Build history of the part. All positions in model axes, mm. A direction names the side the tool comes from. Give positions to 0.01 mm unless a question says otherwise; leave off trailing zeros. Order: outer loops, then holes, each group sorted by start corner. A loop starts at its lowest first (then second) coordinate and runs counter-clockwise, first axis right, second up. Notation, with made-up numbers: M 65.5,43.25 L 95.5,43.25 A16 cw 95.5,59.25 Z; hole C 44,39 d4. An arc over 180 degrees is marked long. Use CSV: the item, a comma, the result in double quotes. Start each with the question number.
Item 1: Two-plate mould, pull along Z, no slides. Class faces 4 (the flat face through (-10.433, 25, 3)), 5 (the flat face through (-12.433, 26, 2)), 6 (the cylindrical face through (-9.357, 35.21, 0.994)), 7 (the flat face through (11, 68, -1.834)): pulls with the +Z half, pulls with the -Z half, needs draft (parallel to the pull), parting line crosses it, or undercut.
Item 2: Which spindle directions (+Z, -Z, +X, -X, +Y, -Y) get a long thin tool onto all of the face, cutting with end or side? Do faces 1 (the flat face through (-2.933, 79, -12)), 2 (the cylindrical face through (2.27, 72.71, 10.75)), 3 (the flat face through (2.067, 79, -12)). Say none if no direction does.
Item 3: Band-saw the part on D-D on z = -11. Write the cut outline in (x, y), plus the area to 3 significant figures.
Item 4: Band-saw the part on A-A on y = 32. Write the cut outline in (x, z).
Item 5: Wall check: line 1 along X through (y, z) = (19, 3.5); line 2 along Z through (x, y) = (8.75, 30); line 3 along Z through (x, y) = (4.5, 45.5). Give the ranges that are in metal, low to high.
Item 6: Band-saw the part on B-B on y = 17.5. Write the cut outline in (x, z).
Item 7: Band-saw the part on C-C on x = -4.5. Write the cut outline in (y, z).
Item 8: Pin check, flat tips, straight feed: P1, Ø3, axis at x = 6, z = 8.5, coming from the -Y side; P2, Ø2, axis at x = 7.5, z = -8.5, coming from the -Y side; P3, Ø7, axis at x = 0.5, z = 1.5, coming from the -Y side; P4, Ø1.5, axis at y = 73.5, z = 2.5, coming from the +X side. Stop position of each tip, or through.
from build123d import *

# Parameters (mm, degrees)
SKETCH1_W            = 24
SKETCH1_H            = 24
SKETCH1_W_2          = 20
SKETCH1_H_2          = 20
BOSS_EXTRUDE1_DEPTH  = 50
FILLET1_R            = 1
FILLET2_R            = 1
BOSS_EXTRUDE7_START  = 2
BOSS_EXTRUDE7_DEPTH  = 2
SKETCH9_R            = 9
BOSS_EXTRUDE9_DEPTH  = 30
SKETCH10_R           = 7
CUT_EXTRUDE1_DEPTH   = 34
SKETCH11_R           = 9
SKETCH11_R_2         = 7
BOSS_EXTRUDE10_DEPTH = 40
BOSS_EXTRUDE12_DEPTH = 1
FILLET3_R            = 1
SKETCH15_R           = 9
BOSS_EXTRUDE13_DEPTH = 2
BOSS_EXTRUDE15_DEPTH = 1
FILLET5_R            = 1
SKETCH18_W           = 5
SKETCH18_H           = 5
BOSS_EXTRUDE16_DEPTH = 1


with BuildPart() as part:
    # Sketch1 → Boss-Extrude1 (new body)
    with BuildSketch(Plane(origin=(0, 0, 0), x_dir=(1, 0, 0), z_dir=(0, 1, 0))):
        with Locations((-0.433212996, -2.166064982)):
            Rectangle(SKETCH1_W, SKETCH1_H)
        with Locations((-0.433212996, -2.166064982)):
            Rectangle(SKETCH1_W_2, SKETCH1_H_2, mode=Mode.SUBTRACT)
    extrude(amount=BOSS_EXTRUDE1_DEPTH)

    # Fillet1
    fillet1_edges = [part.edges().sort_by_distance(p)[0] for p in [
        (-10.433212996, 25, -7.833935018),
        (11.566787004, 25, -9.833935018),
        (11.566787004, 25, 14.166064982),
        (-12.433212996, 25, 14.166064982),
    ]]
    fillet(fillet1_edges, radius=FILLET1_R)

    # Fillet2
    fillet2_edges = [part.edges().sort_by_distance(p)[0] for p in [
        (-12.433212996, 25, -9.833935018),
    ]]
    fillet(fillet2_edges, radius=FILLET2_R)

    # Sketch8 → Boss-Extrude7 (add)
    with BuildSketch(Plane(origin=(0, 50, 0), x_dir=(1, 0, 0), z_dir=(0, 1, 0)).offset(BOSS_EXTRUDE7_START)):
        with BuildLine():
            Line((10.566787004, 9.833935018), (-11.433212996, 9.833935018))
            ThreePointArc((-11.433212996, 9.833935018), (-12.140319778, 9.541041799), (-12.433212996, 8.833935018))
            Line((-12.433212996, 8.833935018), (-12.433212996, -13.166064982))
            ThreePointArc((-12.433212996, -13.166064982), (-12.140319778, -13.873171763), (-11.433212996, -14.166064982))
            Line((-11.433212996, -14.166064982), (10.566787004, -14.166064982))
            ThreePointArc((10.566787004, -14.166064982), (11.273893785, -13.873171763), (11.566787004, -13.166064982))
            Line((11.566787004, -13.166064982), (11.566787004, 8.833935018))
            ThreePointArc((11.566787004, 8.833935018), (11.273893785, 9.541041799), (10.566787004, 9.833935018))
        make_face()
    extrude(amount=-BOSS_EXTRUDE7_DEPTH)

    # Sketch9 → Boss-Extrude9 (add)
    with BuildSketch(Plane.XZ.offset(-50)):
        with Locations(Location((-0.433212996, 2.166064982, 0), (0, 0, 90))):
            Circle(SKETCH9_R)
    extrude(amount=BOSS_EXTRUDE9_DEPTH)

    # Sketch10 → Cut-Extrude1 (cut)
    with BuildSketch(Plane.XZ.offset(-20)):
        with Locations(Location((-0.433212996, 2.166064982, 0), (0, 0, 270))):
            Circle(SKETCH10_R)
    extrude(amount=-CUT_EXTRUDE1_DEPTH, mode=Mode.SUBTRACT)

    # Sketch11 → Boss-Extrude10 (add)
    with BuildSketch(Plane(origin=(0, 52, 0), x_dir=(1, 0, 0), z_dir=(0, 1, 0))):
        with Locations(Location((-0.433212996, -2.166064982, 0), (0, 0, 270))):
            Circle(SKETCH11_R)
        with Locations(Location((-0.433212996, -2.166064982, 0), (0, 0, 90))):
            Circle(SKETCH11_R_2, mode=Mode.SUBTRACT)
    extrude(amount=BOSS_EXTRUDE10_DEPTH)

    # Sketch14 → Boss-Extrude12 (add, symmetric)
    with BuildSketch(Plane(origin=(0, 68, 0), x_dir=(1, 0, 0), z_dir=(0, 1, 0))):
        with BuildLine():
            ThreePointArc((-8.495470745, -6.166064982), (-9.433212996, -2.166064982), (-8.495470745, 1.833935018))
            Line((-8.495470745, 1.833935018), (-15.433212996, 1.833935018))
            Line((-15.433212996, 1.833935018), (-15.433212996, -6.166064982))
            Line((-15.433212996, -6.166064982), (-8.495470745, -6.166064982))
        make_face()
        with BuildLine():
            Line((14.566787004, 1.833935018), (7.629044752, 1.833935018))
            ThreePointArc((7.629044752, 1.833935018), (8.329215883, -0.111840035), (8.566787004, -2.166064982))
            ThreePointArc((8.566787004, -2.166064982), (8.329215883, -4.220289929), (7.629044752, -6.166064982))
            Line((7.629044752, -6.166064982), (14.566787004, -6.166064982))
            Line((14.566787004, -6.166064982), (14.566787004, 1.833935018))
        make_face()
    extrude(amount=BOSS_EXTRUDE12_DEPTH, both=True)

    # Fillet3
    fillet3_edges = [part.edges().sort_by_distance(p)[0] for p in [
        (-15.433212996, 68, -1.833935018),
        (-15.433212996, 68, 6.166064982),
        (14.566787004, 68, 6.166064982),
        (14.566787004, 68, -1.833935018),
    ]]
    fillet(fillet3_edges, radius=FILLET3_R)

    # Sketch15 → Boss-Extrude13 (add)
    with BuildSketch(Plane(origin=(0, 92, 0), x_dir=(1, 0, 0), z_dir=(0, 1, 0))):
        with Locations(Location((-0.433212996, -2.166064982, 0), (0, 0, 270))):
            Circle(SKETCH15_R)
    extrude(amount=BOSS_EXTRUDE13_DEPTH)

    # Sketch17 → Boss-Extrude15 (add, symmetric)
    with BuildSketch(Plane(origin=(0, 79, 0), x_dir=(1, 0, 0), z_dir=(0, 1, 0))):
        with BuildLine():
            Line((2.066787004, 17.833935018), (-2.933212996, 17.833935018))
            Line((-2.933212996, 17.833935018), (-2.933212996, 6.479743251))
            ThreePointArc((-2.933212996, 6.479743251), (-0.433212996, 6.833935018), (2.066787004, 6.479743251))
            Line((2.066787004, 6.479743251), (2.066787004, 17.833935018))
        make_face()
    extrude(amount=BOSS_EXTRUDE15_DEPTH, both=True)

    # Fillet5
    fillet5_edges = [part.edges().sort_by_distance(p)[0] for p in [
        (2.066787004, 79, -17.833935018),
        (-2.933212996, 79, -17.833935018),
    ]]
    fillet(fillet5_edges, radius=FILLET5_R)

    # Sketch18 → Boss-Extrude16 (add, symmetric)
    with BuildSketch(Plane(origin=(0, 94, 0), x_dir=(1, 0, 0), z_dir=(0, 1, 0))):
        with Locations((-0.433212996, -2.166064982)):
            Rectangle(SKETCH18_W, SKETCH18_H)
    extrude(amount=BOSS_EXTRUDE16_DEPTH, both=True)


solid = part.part
Model answer:
1,face 4,"undercut"
1,face 5,"needs draft"
1,face 6,"undercut"
1,face 7,"pulls with the -Z half"
2,face 1,"-Z, -X, +Y"
2,face 2,"none"
2,face 3,"-Z, +X, +Y"
3,outline,"M -2.93,78 L 2.07,78 L 2.07,80 L -2.93,80 Z"
3,area,"10.0 mm^2"
4,outline,"M -12.43,-8.83 A1 ccw -11.43,-9.83 L 10.57,-9.83 A1 ccw 11.57,-8.83 L 11.57,13.17 A1 ccw 10.57,14.17 L -11.43,14.17 A1 ccw -12.43,13.17 Z; C -0.43,2.17 d18; hole M -10.43,-6.83 A1 ccw -9.43,-7.83 L 9.57,-7.83 L 9.57,12.17 L -10.43,12.17 Z; hole C -0.43,2.17 d14"
5,line 1,"x = -12.43 to -10.43, 9.57 to 11.57"
5,line 2,"z = -9.83 to -7.83, 12.17 to 14.17"
5,line 3,"z = -9.83 to -7.83, -5.36 to -2.8, 7.13 to 9.69, 12.17 to 14.17"
6,outline,"M -12.43,-8.83 A1 ccw -11.43,-9.83 L 10.57,-9.83 A1 ccw 11.57,-8.83 L 11.57,13.17 A1 ccw 10.57,14.17 L -11.43,14.17 A1 ccw -12.43,13.17 Z; hole M -10.43,-6.83 A1 ccw -9.43,-7.83 L 9.57,-7.83 L 9.57,12.17 L -10.43,12.17 Z"
7,outline,"M 0,-9.83 L 52,-9.83 L 52,-5.86 L 94,-5.86 L 94,10.19 L 52,10.19 L 52,14.17 L 0,14.17 L 0,12.17 L 50,12.17 L 50,10.19 L 20,10.19 L 20,7.86 L 92,7.86 L 92,-3.53 L 20,-3.53 L 20,-5.86 L 50,-5.86 L 50,-7.83 L 0,-7.83 Z"
8,P1,"stops at y = 20"
8,P2,"stops at y = 0"
8,P3,"stops at y = 92"
8,P4,"stops at x = 8.57"
